Autodesk Inventor part; units mm, degrees
ref_plane "YZ Plane" through (0, 0, 0) normal (1, 0, 0) x (0, 1, 0)
ref_plane "XZ Plane" through (0, 0, 0) normal (0, 1, 0) x (-1, 0, 0)
ref_plane "XY Plane" through (0, 0, 0) normal (0, 0, 1) x (1, 0, 0)
sketch "Sketch1" plane through (0, 0, 0) normal (0, 0, 1) x (1, 0, 0)
  line L0 (8, 0) -> (86, 0)
  line L1 (94, 8) -> (94, 24)
  line L2 (86, 32) -> (8, 32)
  line L3 (0, 24) -> (0, 8)
  arc A0 (8, 32) -> (0, 24) centre (8, 24) ccw
  arc A1 (94, 24) -> (86, 32) centre (86, 24) ccw
  arc A2 (86, 0) -> (94, 8) centre (86, 8) ccw
  arc A3 (0, 8) -> (8, 0) centre (8, 8) ccw
  circle A4 centre (51, 20) radius 5
  point P0 (0, 0)
  point P1 (94, 32)
  point P2 (94, 0)
  point P3 (0, 32)
  dimension "d0" = 94
  dimension "d1" = 32
  dimension "d2" = 8
  dimension "d3" = 8
  dimension "d6" = 10
extrude "Extrusion1" add sketch "Sketch1" along normal blind 4 contours A3 L3 A0 L2 A1 L1 A2 L0 | A4
properties part number "PistonFeederHeadInnerMini" material "Stainless Steel"
Verification items for the finished model (mm, model axes). Coordinates: 2 decimals unless noted, no trailing zeros. Order: outer loops, then holes, each group sorted by start corner. A loop starts at its lowest first (then second) coordinate and runs counter-clockwise, first axis right, second up. Notation, with made-up numbers: (75.5, 29) -> (95.5, 29) arc R8 cw to (95.5, 44) -> close; hole circle Ø4 at (76.5, 51). An arc over 180 degrees is marked (long way). Put each result on its own line as item: value. Start each with the question number.
1) Cross-section at C-C (y = 30). Enter the section's corners in (x, z), plus the area to 3 significant figures.
2) Go/stop test with a flat-tipped pin: pin 1 (1.5 mm diameter, centred on x = 79, z = 3.5, fed in from -Y). Record where the tip stops, or that it passes through.
3) Cross-section at B-B (y = 3). Enter the section's corners in (x, z) (3 decimals), plus the area to 3 significant figures.
4) Material ranges on L1, parallel to X at y = 3, z = 2.45 (3 decimals); L2, parallel to X at y = 26.5, z = 1.55; L3, parallel to Y at x = 88, z = 2.5, recorded low to high.
5) Cross-section at A-A (z = 2.6). Enter the section's corners in (x, y), plus the area to 3 significant figures.
Geometry check:
1. outline: (2.71, 0) -> (91.29, 0) -> (91.29, 4) -> (2.71, 4) -> close
1. area: 354 mm^2
2. pin 1: stops at y = 0
3. outline: (1.755, 0) -> (92.245, 0) -> (92.245, 4) -> (1.755, 4) -> close
3. area: 362 mm^2
4. L1: x = 1.755 to 92.245
4. L2: x = 0.4 to 93.6
4. L3: y = 0.25 to 31.75
5. outline: (0, 8) arc R8 ccw to (8, 0) -> (86, 0) arc R8 ccw to (94, 8) -> (94, 24) arc R8 ccw to (86, 32) -> (8, 32) arc R8 ccw to (0, 24) -> close
5. area: 2,950 mm^2
